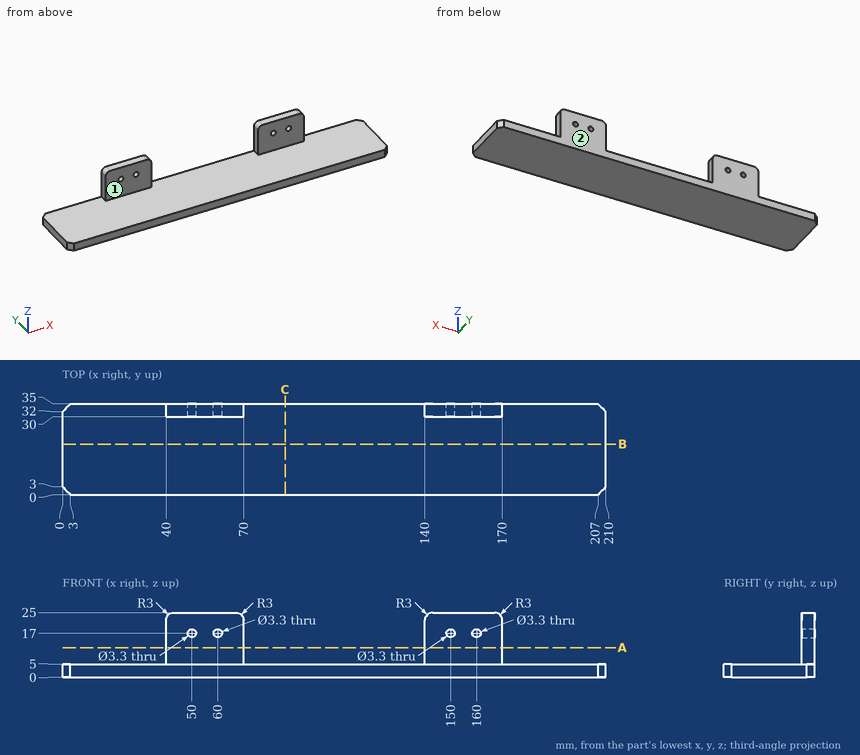
Can you work these out from the drawing? Everything is in mm from the part's minimum corner. A direction names the side the tool comes from. Coordinates: 2 decimals unless noted, no trailing zeros. Loops run counter-clockwise (first coordinate to the right, second up) from the corner with the lowest first, then second, coordinate; pieces in that order, holes last.
1. I need wall thicknesses on L1, parallel to X at y = 31.15, z = 17; L2, parallel to Z at x = 150, y = 31.7; L3, parallel to X at y = 30.5, z = 14. Which ranges of each line are inside material? Lowest first, please.
2. Imagine slicing it at B-B, the plane y = 19.5. Please give me the cut outline in (x, z).
3. For P1, Ø4.5, axis at x = 160, z = 17, coming from the +Y side; P2, Ø5.5, axis at x = 60, z = 17, coming from the -Y side; P3, Ø5.5, axis at y = 32, z = 11, coming from the +X side; P4, Ø1.5, axis at y = 33, z = 15.5, coming from the -X side, each with a flat end and sliding along its axis, tell me the tip position at first contact or that it passes through.
4. Imagine slicing it at C-C, the plane x = 86. Please give me the cut outline in (y, z).
5. For the marked faces 1 and 2, which set-ups out of +Z, -Z, +X, -X, +Y, -Y let a thin tool reach every point of the face, with its end or its side?
6. Imagine slicing it at A-A, the plane z = 11.5. Please give me the cut outline in (x, y).
Taken from the geometry:
1. L1: x = 40 to 48.35, 51.65 to 58.35, 61.65 to 70, 140 to 148.35, 151.65 to 158.35, 161.65 to 170
1. L2: z = 0 to 15.35, 18.65 to 25
1. L3: x = 40 to 70, 140 to 170
2. outline: (0, 0) - (210, 0) - (210, 5) - (0, 5) - close
3. P1: stops at y = 35
3. P2: stops at y = 30
3. P3: stops at x = 170
3. P4: stops at x = 40
4. outline: (0, 0) - (35, 0) - (35, 5) - (0, 5) - close
5. face 1: +Z, +X, -X, -Y
5. face 2: +Z, -Z, +X, -X, +Y
6. outline: (40, 30) - (70, 30) - (70, 35) - (40, 35) - close; (140, 30) - (170, 30) - (170, 35) - (140, 35) - close
